Verification items for the finished model (mm, model axes). A direction names the side the tool comes from. Give positions to 0.01 mm unless a question says otherwise; leave off trailing zeros. Loops run counter-clockwise (first coordinate to the right, second up) from the corner with the lowest first, then second, coordinate; pieces in that order, holes last. Notation, with made-up numbers: (8.25, 57) - (41.25, 57) arc R19 cw to (41.25, 91) - close; hole circle Ø2 at (55.5, 65.25). An arc over 180 degrees is marked (long way). One line per question, with ' | ' between items. Start each with the question number.
1. Section check C-C, the plane z = 1.35. Enter the section's corners in (x, y), then the cut area to 3 significant figures.
2. Section check B-B, the plane z = 3.15. Enter the section's corners in (x, y).
3. Section check A-A, the plane x = 2.5. Enter the section's corners in (y, z), then the cut area to 3 significant figures.
4. Tool access check on faces 1 (the face through (0, 17.1, 1)), 2 (the face through (0, 16, 1.8)), 3 (the face through (0, -16, 1.8)), 4 (the face through (0, -17.1, 1)). Record the directions out of +Z, -Z, +X, -X, +Y, -Y that give a thin tool (end or side, any length) a straight path to the whole face; none if there is none.
5. Thickness scan on line 1 along Z through (x, y) = (-4, -17); line 2 along Y through (x, z) = (-1, 5.1); line 3 along X through (y, z) = (10, 4.4). Record the ranges inside material, lowest first. Write a range as from..to.
6. Depth check by flat-ended pin: pin 1 Ø2 at (x, z) = (1.5, 4) entering from -Y; pin 2 Ø1.6 at (y, z) = (18, 1.5) entering from -X; pin 3 Ø1.4 at (x, z) = (0.5, 1) entering from -Y. Enter the tip coordinate at first touch or a pass-through.
from build123d import *

# Parameters (mm, degrees)
SKETCH1_W   = 16.5
SKETCH1_H   = 34.2
INT_2_DEPTH = 1.8
SKETCH2_W   = 16.5
SKETCH2_H   = 31.2
EXT_DEPTH   = 3.5
SKETCH3_W   = 5.3
SKETCH3_H   = 37.5
TOP_DEPTH   = 3
FILLET1_R   = 1


with BuildPart() as part:
    # Sketch1 → Int 2 (new body)
    with BuildSketch(Plane.XY):
        Rectangle(SKETCH1_W, SKETCH1_H)
    extrude(amount=INT_2_DEPTH)

    # Sketch2 → Ext (add)
    with BuildSketch(Plane.XY.offset(1.8)):
        Rectangle(SKETCH2_W, SKETCH2_H)
    extrude(amount=EXT_DEPTH)

    # Sketch3 → Top (add)
    with BuildSketch(Plane(origin=(8.25, 0, 0), x_dir=(0, 0, -1), z_dir=(1, 0, 0))):
        with Locations((-2.65, 0)):
            Rectangle(SKETCH3_W, SKETCH3_H)
    extrude(amount=TOP_DEPTH)

    # Fillet1
    fillet1_edges = [part.edges().sort_by_distance(p)[0] for p in [
        (11.25, 0, 0),
        (11.25, 18.75, 2.65),
        (11.25, 0, 5.3),
        (11.25, -18.75, 2.65),
    ]]
    fillet(fillet1_edges, radius=FILLET1_R)


solid = part.part
Results list:
1) outline: (-8.25, -17.1) - (8.25, -17.1) - (8.25, -18.75) - (10.25, -18.75) arc R1 ccw to (11.25, -17.75) - (11.25, 17.75) arc R1 ccw to (10.25, 18.75) - (8.25, 18.75) - (8.25, 17.1) - (-8.25, 17.1) - close | area: 676 mm²
2) outline: (-8.25, -15.6) - (8.25, -15.6) - (8.25, -18.75) - (10.25, -18.75) arc R1 ccw to (11.25, -17.75) - (11.25, 17.75) arc R1 ccw to (10.25, 18.75) - (8.25, 18.75) - (8.25, 15.6) - (-8.25, 15.6) - close
3) outline: (-17.1, 0) - (17.1, 0) - (17.1, 1.8) - (15.6, 1.8) - (15.6, 5.3) - (-15.6, 5.3) - (-15.6, 1.8) - (-17.1, 1.8) - close | area: 171 mm²
4) face 1: +Z, -Z, -X, +Y | face 2: +Z, -X, +Y | face 3: +Z, -X, -Y | face 4: +Z, -Z, -X, -Y
5) line 1: 0..1.8 | line 2: -15.6..15.6 | line 3: -8.25..11.24
6) pin 1: y = -15.6 | pin 2: x = 8.25 | pin 3: y = -17.1
